Source: CAD feature listing. Evaluate the final solid. Frame: model axes, mm. A direction names the side the tool comes from. Coordinates: 2 decimals unless noted, no trailing zeros. Loops run counter-clockwise (first coordinate to the right, second up) from the corner with the lowest first, then second, coordinate; pieces in that order, holes last. Notation, with made-up numbers: (-5.5, 10) - (25.5, 10) arc R9 cw to (25.5, 19) - close; hole circle Ø3 at (53, 17.25). An arc over 180 degrees is marked (long way). Write item = value, one per line. Start each with the question number.
from build123d import *

# Parameters (mm, degrees)
F1_DEPTH  = 12
F3_DEPTH  = 10.5
F4_DEPTH  = 25
F7_DEPTH  = 25
F9_DEPTH  = 25
F12_DEPTH = 8
F13_W     = 1
F13_H     = 20
F13_H_2   = 18.9817659557
F14_DEPTH = 12.5


with BuildPart() as f1:
    # F0 (on Top) → F1 (new body)
    with BuildSketch(Plane.XY):
        with BuildLine():
            Line((11.25, 4), (11.25, 0))
            Line((11.25, 0), (11.25, -4))
            Line((11.25, -4), (10.5148704224, -4))
            ThreePointArc((10.5148704224, -4), (6.3860198872, -9.2618167764), (0, -11.25))
            Line((0, -11.25), (0, -13.25))
            ThreePointArc((0, -13.25), (9.3691648507, -9.3691648507), (13.25, 0))
            ThreePointArc((13.25, 0), (9.3691648507, 9.3691648507), (0, 13.25))
            Line((0, 13.25), (0, 11.25))
            ThreePointArc((0, 11.25), (6.3860198872, 9.2618167764), (10.5148704224, 4))
            Line((10.5148704224, 4), (11.25, 4))
        make_face()
        with BuildLine():
            Line((10.5148704224, -4), (6.0466933112, -4))
            ThreePointArc((6.0466933112, -4), (3.4323825544, -6.3860198872), (0, -7.25))
            Line((0, -7.25), (0, -11.25))
            ThreePointArc((0, -11.25), (6.3860198872, -9.2618167764), (10.5148704224, -4))
        make_face()
        with BuildLine():
            Line((11.25, 0), (7.25, 0))
            ThreePointArc((7.25, 0), (6.9426589469, -2.0885369872), (6.0466933112, -4))
            Line((6.0466933112, -4), (10.5148704224, -4))
            ThreePointArc((10.5148704224, -4), (11.0646914158, -2.0334954817), (11.25, 0))
        make_face()
        with BuildLine():
            ThreePointArc((6.0466933112, 4), (6.9426589469, 2.0885369872), (7.25, 0))
            Line((7.25, 0), (11.25, 0))
            ThreePointArc((11.25, 0), (11.0646914158, 2.0334954817), (10.5148704224, 4))
            Line((10.5148704224, 4), (6.0466933112, 4))
        make_face()
        with BuildLine():
            ThreePointArc((10.5148704224, 4), (11.0646914158, 2.0334954817), (11.25, 0))
            Line((11.25, 0), (11.25, 4))
            Line((11.25, 4), (10.5148704224, 4))
        make_face()
        with BuildLine():
            Line((11.25, -4), (11.25, 0))
            ThreePointArc((11.25, 0), (11.0646914158, -2.0334954817), (10.5148704224, -4))
            Line((10.5148704224, -4), (11.25, -4))
        make_face()
        with BuildLine():
            ThreePointArc((0, 7.25), (3.4323825544, 6.3860198872), (6.0466933112, 4))
            Line((6.0466933112, 4), (10.5148704224, 4))
            ThreePointArc((10.5148704224, 4), (6.3860198872, 9.2618167764), (0, 11.25))
            Line((0, 11.25), (0, 7.25))
        make_face()
    extrude(amount=F1_DEPTH)

    # F2 (on Right) → F3 (cut)
    with BuildSketch(Plane.YZ):
        with BuildLine():
            ThreePointArc((4.2, 6), (-2.969848481, 8.969848481), (0, 1.8))
            ThreePointArc((0, 1.8), (2.969848481, 3.030151519), (4.2, 6))
        make_face()
        with BuildLine():
            ThreePointArc((2.1, 6), (1.4849242405, 4.5150757595), (0, 3.9))
            ThreePointArc((0, 3.9), (-1.4849242405, 7.4849242405), (2.1, 6))
        make_face(mode=Mode.SUBTRACT)
        with BuildLine():
            ThreePointArc((2.1, 6), (-1.4849242405, 7.4849242405), (0, 3.9))
            ThreePointArc((0, 3.9), (1.4849242405, 4.5150757595), (2.1, 6))
        make_face()
    extrude(amount=F3_DEPTH, mode=Mode.SUBTRACT)

    # F2 (on Right) → F4 (cut)
    with BuildSketch(Plane.YZ):
        with BuildLine():
            ThreePointArc((2.1, 6), (-1.4849242405, 7.4849242405), (0, 3.9))
            ThreePointArc((0, 3.9), (1.4849242405, 4.5150757595), (2.1, 6))
        make_face()
    extrude(amount=F4_DEPTH, mode=Mode.SUBTRACT)

    # F6 (on face) → F7 (cut)
    with BuildSketch(Plane(origin=(0, 0, 0), x_dir=(0, -1, 0), z_dir=(-1, 0, 0))):
        with BuildLine():
            ThreePointArc((12.05, 6), (10.25, 7.8), (8.45, 6))
            Line((8.45, 6), (12.05, 6))
        make_face()
        with BuildLine():
            Line((12.05, 6), (8.45, 6))
            ThreePointArc((8.45, 6), (10.25, 4.2), (12.05, 6))
        make_face()
    extrude(amount=-F7_DEPTH, mode=Mode.SUBTRACT)

    # F8 (on face) → F9 (cut)
    with BuildSketch(Plane(origin=(0, 0, 0), x_dir=(0, -1, 0), z_dir=(-1, 0, 0))):
        with BuildLine():
            Line((-12.05, 6), (-8.45, 6))
            ThreePointArc((-8.45, 6), (-10.25, 7.8), (-12.05, 6))
        make_face()
        with BuildLine():
            ThreePointArc((-12.05, 6), (-10.25, 4.2), (-8.45, 6))
            Line((-8.45, 6), (-12.05, 6))
        make_face()
    extrude(amount=-F9_DEPTH, mode=Mode.SUBTRACT)

    # F11 (on offset) → F12 (cut)
    with BuildSketch(Plane.YZ.offset(13)):
        Polygon((-7.6, 4.3256842194), (-7.6, 6), (-7.6, 7.6743157806), (-10.5, 9.3486315613), (-13.4, 7.6743157806), (-13.4, 4.3256842194), (-10.5, 2.6513684387), align=None)
        Polygon((7.6, 7.6743157806), (7.6, 6), (7.6, 4.3256842194), (10.5, 2.6513684387), (13.4, 4.3256842194), (13.4, 7.6743157806), (10.5, 9.3486315613), align=None)
    extrude(amount=-F12_DEPTH, mode=Mode.SUBTRACT)

    # F13 (on Top) → F14 (cut, symmetric)
    with BuildSketch(Plane.XY):
        with Locations((0.5, 10)):
            Rectangle(F13_W, F13_H)
        with Locations((0.5, -9.4908829778)):
            Rectangle(F13_W, F13_H_2)
    extrude(amount=F14_DEPTH, both=True, mode=Mode.SUBTRACT)


solid = f1.part
Item 1: Draft query along Y for faces 1 (the flat face through (8, 0, 12)), 2 (the flat face through (7.317, 9.07, 8.523)), 3 (the flat face through (8, -7.6, 6)). Return one class per face: released by +Y, released by -Y, zero draft, split by the parting line, or undercut.
Item 2: Cut plane B-B (y = -2.5). Return the cut outline in (x, z).
Item 3: Material intervals for L1, parallel to Y at x = 9.4, z = 6; L2, parallel to Z at x = 8.6, y = 0; L3, parallel to Y at x = 3.9, z = 6, sorted ascending. Write a range as [from, to].
Item 4: Cut plane A-A (x = 2.75). Return the cut outline in (y, z).
Item 5: Reachability of faces 4 (the flat face through (8, 0, 0)), 5 (the flat face through (5, 8, 6)), 6 (the flat face through (8, 7.6, 6)) from +Z, -Z, +X, -X, +Y, -Y: full face, straight path, thin tool, end or side. Return the list, or none.
Item 6: Cut plane C-C (x = 12.25). Return the cut outline in (y, z), then the cut area to 3 significant figures.
Item 7: First-contact query: pin 1 (6 mm diameter, centred on y = -10.25, z = 6, fed in from +X); pin 2 (1.7 mm diameter, centred on x = 7.5, z = 6.5, fed in from -Y); pin 3 (1 mm diameter, centred on x = 7, z = 8, fed in from -Y). Flat tips, straight axial feed; report the tip coordinate or a pass-through.
Responses:
q1.face_1 = zero draft
q1.face_2 = undercut
q1.face_3 = released by -Y
q2.outline = (6.81, 0) - (13.01, 0) - (13.01, 12) - (6.81, 12) - (6.81, 9.37) - (10.5, 9.37) - (10.5, 2.63) - (6.81, 2.63) - close
q3.L1 = [-7.6, -4.2], [4.2, 7.6]
q3.L2 = [0, 1.8], [10.2, 12]
q3.L3 = [-12.66, -12.05], [-8.45, -6.11], [6.11, 8.45], [12.05, 12.66]
q4.outline = (-12.96, 0) - (-6.71, 0) - (-6.71, 12) - (-12.96, 12) - close; (6.71, 0) - (12.96, 0) - (12.96, 12) - (6.71, 12) - close; hole circle Ø3.6 at (-10.25, 6); hole circle Ø3.6 at (10.25, 6)
q5.face_4 = -Z, +X, -X, +Y, -Y
q5.face_5 = +X
q5.face_6 = +X, +Y
q6.outline = (-5.05, 0) - (5.05, 0) - (5.05, 12) - (-5.05, 12) - close; hole circle Ø4.2 at (0, 6)
q6.area = 107 mm2
q7.pin_1 = 11.09
q7.pin_2 = -7.6
q7.pin_3 = -9.03
